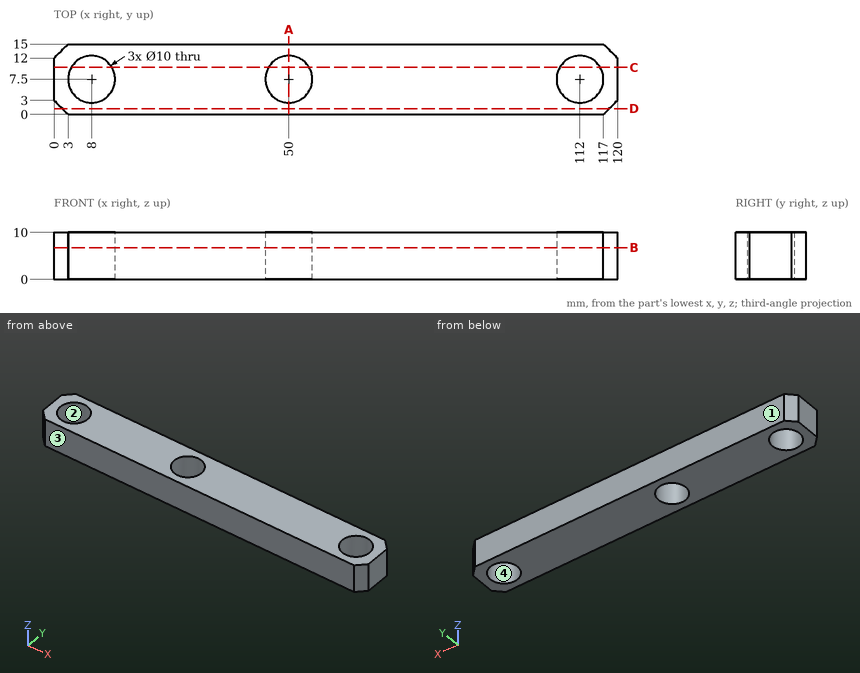
Geometry: see drawing. Coordinates: mm, zero at the bounding-box minimum. Round coordinates to 2 decimals unless told otherwise and drop trailing zeros. Loops run counter-clockwise (first coordinate to the right, second up) from the corner with the lowest first, then second, coordinate; pieces in that order, holes last. Notation, with made-up numbers: (-8, 4.5) - (7, 4.5) arc R31 ccw to (7, 38.5) - close; hole circle Ø5 at (-7.5, 49). An arc over 180 degrees is marked (long way). Use CSV: the item, a comma, the result in double quotes.
Q1. Ray query, line 1 along Y through (x, z) = (50, 3.75); line 2 along X through (y, z) = (5.75, 1.5); line 3 along Y through (x, z) = (51.5, 7.75). Return the intervals inside material, ascending.
Reported:
line 1,"0 to 2.5, 12.5 to 15"
line 2,"0 to 3.32, 12.68 to 45.32, 54.68 to 107.32, 116.68 to 120"
line 3,"0 to 2.73, 12.27 to 15"
Q2. Mould query, pull axis Y, two halves, no side actions, for the marked faces 1, 2, 3 and 4. Classes: pulls with the +Y half, pulls with the -Y half, needs draft (parallel to the pull), parting line crosses it, or undercut.
Reported:
face 1,"pulls with the +Y half"
face 2,"undercut"
face 3,"pulls with the -Y half"
face 4,"undercut"
Q3. Pin query (flat end, axial travel): pin 1 Ø9 at (x, y) = (112, 7.5) entering from -Z. Return the tip coordinate at first contact, or that it passes through.
Reported:
pin 1,"through"
Q4. Section query D-D, the plane y = 1.25. Output: boundary loops of the cut face in (x, z).
Reported:
outline,"(1.75, 0) - (118.25, 0) - (118.25, 10) - (1.75, 10) - close"
Q5. Section query A-A, the plane x = 50. Output: boundary loops of the cut face in (y, z), then the cut area to 3 significant figures.
Reported:
outline,"(0, 0) - (2.5, 0) - (2.5, 10) - (0, 10) - close; (12.5, 0) - (15, 0) - (15, 10) - (12.5, 10) - close"
area,"50.0 mm^2"
Q6. Section query C-C, the plane y = 10. Output: boundary loops of the cut face in (x, z), then the cut area to 3 significant figures.
Reported:
outline,"(0, 0) - (3.67, 0) - (3.67, 10) - (0, 10) - close; (12.33, 0) - (45.67, 0) - (45.67, 10) - (12.33, 10) - close; (54.33, 0) - (107.67, 0) - (107.67, 10) - (54.33, 10) - close; (116.33, 0) - (120, 0) - (120, 10) - (116.33, 10) - close"
area,"940 mm^2"
Q7. Section query B-B, the plane z = 6.75. Output: boundary loops of the cut face in (x, y).
Reported:
outline,"(0, 3) - (3, 0) - (117, 0) - (120, 3) - (120, 12) - (117, 15) - (3, 15) - (0, 12) - close; hole circle Ø10 at (8, 7.5); hole circle Ø10 at (50, 7.5); hole circle Ø10 at (112, 7.5)"
